For this review, use the dimensioned drawing (mm, ordinates from the lowest corner) and the shaded views. A direction names the side the tool comes from. Give positions to 0.01 mm unless a question says otherwise; leave off trailing zeros. Order: outer loops, then holes, each group sorted by start corner. A loop starts at its lowest first (then second) coordinate and runs counter-clockwise, first axis right, second up. Notation, with made-up numbers: M -38.5,66.5 L -20.5,66.5 A18 cw -20.5,96.5 Z; hole C 27,62 d6. An arc over 180 degrees is marked long. Use CSV: the item, a comma, the result in double quotes. Start each with the question number.
(1) Consider section C-C (x = 60). Write out the cut boundary in (y, z).
(2) Consider section B-B (z = 64). Give the number of separate pieces and of enclosed holes in the cut face, and give its area (3 significant figures).
(3) Tool access review of the marked faces 4, 5 and 6: name each direction out of +Z, -Z, +X, -X, +Y, -Y from which nothing blocks a thin tool from reaching the whole face with its end or side.
(4) Wall thickness on L1, parallel to Z at x = 12, y = 4.5; L2, parallel to X at y = 4.25, z = 13.5; L3, parallel to X at y = 6.75, z = 61: over which ranges is each line inside the solid? List them lowest first. Write a range as from..to.
(5) Clearance check with flat-ended pins moving along their axes: P1, Ø1, axis at y = 13.5, z = 40.5, coming from the +X side; P2, Ø6, axis at x = 22, z = 52, coming from the +Y side; P3, Ø10, axis at x = 12, z = 62, coming from the -Y side; P4, Ø22, axis at x = 68, z = 47, coming from the -Y side. State where each tip first meets the part, or that it passes through.
(6) Draft analysis for pull direction X (two halves, no side actions). For the marked faces 1, 2 and 3, state which applies: pulls with the +X half, pulls with the -X half, needs draft (parallel to the pull), parting line crosses it, or undercut.
(7) Consider section D-D (x = 20). Write out the cut boundary in (y, z).
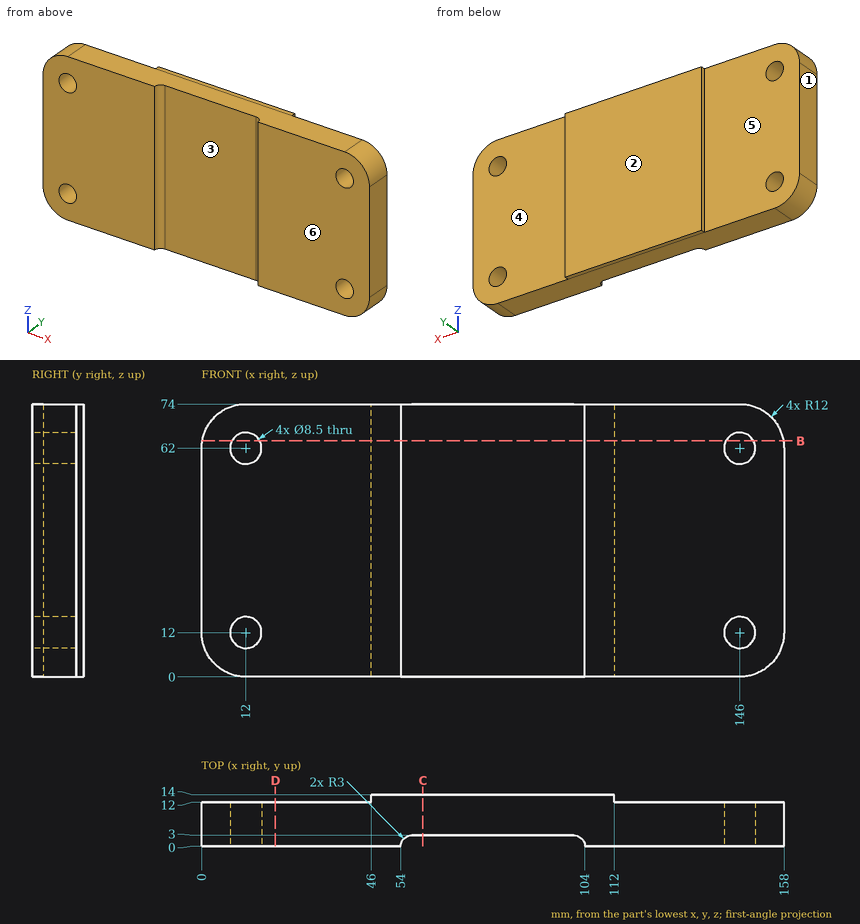
Check result:
1,outline,"M 3,0 L 14,0 L 14,74 L 3,74 Z"
2,separate pieces,"3"
2,enclosed holes,"0"
2,area,"1,700 mm^2"
3,face 4,"+Z, -Z, +X, +Y"
3,face 5,"+Z, -Z, -X, +Y"
3,face 6,"+Z, -Z, +X, -X, -Y"
4,L1,"z = 0..7.75, 16.25..57.75, 66.25..74"
4,L2,"x = 0..8.02, 15.98..142.02, 149.98..158"
4,L3,"x = 0..7.87, 16.13..141.87, 150.13..158"
5,P1,"stops at x = 112"
5,P2,"stops at y = 12"
5,P3,"stops at y = 0"
5,P4,"stops at y = 3"
6,face 1,"pulls with the -X half"
6,face 2,"needs draft"
6,face 3,"undercut"
7,outline,"M 0,0 L 12,0 L 12,74 L 0,74 Z"
